Source: CAD feature listing. Evaluate the final solid. Frame: model axes, mm. Face numbers are marked on the shaded views. A direction names the side the tool comes from. Round coordinates to 2 decimals unless told otherwise and drop trailing zeros. Write each loop counter-clockwise with the first axis right and the second up, starting at its lowest first coordinate (ties: lowest second). Pieces come first, ordered by that corner, then holes.
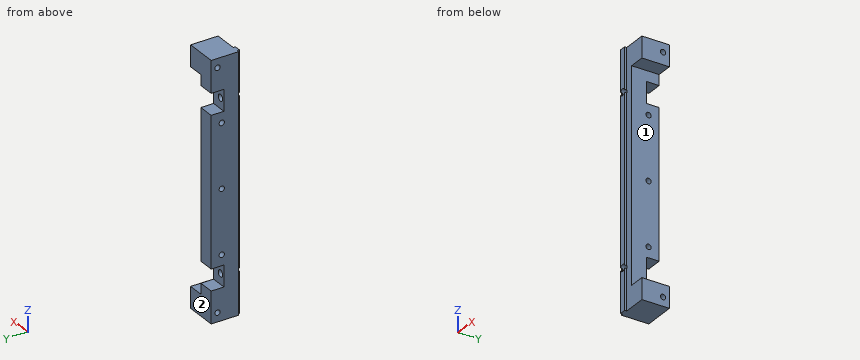
from build123d import *

# Parameters (mm, degrees)
MAIN_DEPTH               = 60
ESQUISSE2_R              = 1.25
HOLESFORMOTORBOARD_DEPTH = 15.95
ESQUISSE4_R              = 1.6
HOLESFORMAKERBEAM_DEPTH  = 15
SKETCH1_W                = 100
SKETCH1_H                = 13
POWERBOARDPINHOLES_DEPTH = 7.45
SKETCH2_R                = 1.25
WINDOWFIXHOLES_DEPTH     = 15.95
SKETCH3_W                = 10
SKETCH3_H                = 6
CUT_EXTRUDE1_DEPTH       = 15.95


with BuildPart() as part:
    # Esquisse1 → Main (new body, symmetric)
    with BuildSketch(Plane.XY):
        Polygon((0, 13), (14.95, 13), (14.95, 0), (3.95, 0), (3.95, -1), (1.05, -1), (1.05, 0), (0, 0), align=None)
    extrude(amount=MAIN_DEPTH, both=True)

    # Esquisse2 → HolesForMotorBoard (cut, through all)
    with BuildSketch(Plane(origin=(14.95, 0, 0), x_dir=(0, 0, -1), z_dir=(1, 0, 0))):
        with Locations((55.75, 10)):
            Circle(ESQUISSE2_R)
        with Locations((-55.75, 10)):
            Circle(ESQUISSE2_R)
    extrude(amount=-HOLESFORMOTORBOARD_DEPTH, mode=Mode.SUBTRACT)

    # Esquisse4 → HolesForMakerBeam (cut, through all)
    with BuildSketch(Plane(origin=(0, -1, 0), x_dir=(-1, 0, 0), z_dir=(0, -1, 0))):
        with Locations((-2.5, -40)):
            Circle(ESQUISSE4_R)
        with Locations((-2.5, 40)):
            Circle(ESQUISSE4_R)
    extrude(amount=-HOLESFORMAKERBEAM_DEPTH, mode=Mode.SUBTRACT)

    # Sketch1 → PowerBoardPinHoles (cut)
    with BuildSketch(Plane(origin=(14.95, 0, 0), x_dir=(0, 0, -1), z_dir=(1, 0, 0))):
        with Locations((0, 6.5)):
            Rectangle(SKETCH1_W, SKETCH1_H)
    extrude(amount=-POWERBOARDPINHOLES_DEPTH, mode=Mode.SUBTRACT)

    # Sketch2 → WindowFixHoles (cut, through all)
    with BuildSketch(Plane.ZY):
        with Locations((0, 8)):
            Circle(SKETCH2_R)
        with Locations((-30, 8)):
            Circle(SKETCH2_R)
        with Locations((30, 8)):
            Circle(SKETCH2_R)
    extrude(amount=-WINDOWFIXHOLES_DEPTH, mode=Mode.SUBTRACT)

    # Sketch3 → Cut-Extrude1 (cut, through all)
    with BuildSketch(Plane.ZY):
        with Locations((-40, 10)):
            Rectangle(SKETCH3_W, SKETCH3_H)
        with Locations((40, 10)):
            Rectangle(SKETCH3_W, SKETCH3_H)
    extrude(amount=-CUT_EXTRUDE1_DEPTH, mode=Mode.SUBTRACT)


solid = part.part
1) Material intervals for line 1 (Z direction, x = 2.5, y = 3); line 2 (Y direction, x = 7, z = -30); line 3 (Z direction, x = 9.25, y = 4.25), sorted ascending.
Taken from the geometry:
line 1: z = -60 to -41.6, -38.4 to 38.4, 41.6 to 60
line 2: y = 0 to 6.75, 9.25 to 13
line 3: z = -60 to -50, 50 to 60
2) Section query C-C on x = 2.5. Return the cut outline in (y, z), then the cut area to 3 significant figures.
Taken from the geometry:
outline: (-1, -60) - (13, -60) - (13, -45) - (7, -45) - (7, -41.6) - (-1, -41.6) - close; (-1, -38.4) - (7, -38.4) - (7, -35) - (13, -35) - (13, 35) - (7, 35) - (7, 38.4) - (-1, 38.4) - close; (-1, 41.6) - (7, 41.6) - (7, 45) - (13, 45) - (13, 60) - (-1, 60) - close; hole circle Ø2.5 at (8, -30); hole circle Ø2.5 at (8, 0); hole circle Ø2.5 at (8, 30); hole circle Ø2.5 at (10, -55.75); hole circle Ø2.5 at (10, 55.75)
area: 1,480 mm2
3) Contact query for flat-ended pins moving along their axis: P1, Ø2, axis at y = 1.5, z = -21, coming from the -X side; P2, Ø3.5, axis at x = 2.5, z = -40, coming from the +Y side; P3, Ø2, axis at y = 3.5, z = -44.5, coming from the +X side; P4, Ø0.8, axis at y = -0.5, z = -54, coming from the +X side. Output: stop coordinate, or through.
Taken from the geometry:
P1: stops at x = 0
P2: stops at y = 7
P3: stops at x = 7.5
P4: stops at x = 3.95
4) Section query A-A on x = 9.5. Return the cut outline in (y, z).
Taken from the geometry:
outline: (0, -60) - (13, -60) - (13, -50) - (0, -50) - close; (0, 50) - (13, 50) - (13, 60) - (0, 60) - close; hole circle Ø2.5 at (10, -55.75); hole circle Ø2.5 at (10, 55.75)
5) Section query B-B on z = -55.75. Return the cut outline in (x, y), then the cut area to 3 significant figures.
Taken from the geometry:
outline: (0, 0) - (1.05, 0) - (1.05, -1) - (3.95, -1) - (3.95, 0) - (14.95, 0) - (14.95, 8.75) - (0, 8.75) - close; (0, 11.25) - (14.95, 11.25) - (14.95, 13) - (0, 13) - close
area: 160 mm2
6) Section query D-D on y = 2. Return the cut outline in (x, z), then the cut area to 3 significant figures.
Taken from the geometry:
outline: (0, -60) - (14.95, -60) - (14.95, -50) - (7.5, -50) - (7.5, 50) - (14.95, 50) - (14.95, 60) - (0, 60) - close; hole circle Ø3.2 at (2.5, -40); hole circle Ø3.2 at (2.5, 40)
area: 1,030 mm2
7) Reachability of the marked faces 1 and 2 from +Z, -Z, +X, -X, +Y, -Y: full face, straight path, thin tool, end or side. Return the list, or none.
Taken from the geometry:
face 1: +X, +Y, -Y
face 2: +Z, -Z, +X, -X, +Y
